Input: dimensioned drawing with shaded views. Units: mm. Origin: part minimum x, y, z. A direction names the side the tool comes from. Round coordinates to 2 decimals unless told otherwise and drop trailing zeros. Write each loop counter-clockwise with the first axis right and the second up, starting at its lowest first coordinate (ties: lowest second). Pieces come first, ordered by that corner, then holes. Notation, with made-up numbers: M 36,28 L 87,28 A12 cw 87,45 Z; hole C 22.5,63.5 d3. An arc over 180 degrees is marked long. Answer in a Markdown table with one row per item. Add a question column.
Item 1: Cut plane C-C on y = 2.25. Return loops of the section in (x, z), and give its area (3 significant figures).
Item 2: Mould query, pull axis Z, two halves, no side actions, for the marked faces 1, 2 and 3. Classes: released by +Z, released by -Z, zero draft, split by the parting line, or undercut.
Item 3: Cut plane A-A on z = 10. Return loops of the section in (x, y).
Item 4: Cut plane D-D on x = 12.5. Return loops of the section in (y, z).
Item 5: Set-up query: the marked faces 4 and 5. Return all of +Z, -Z, +X, -X, +Y, -Y with unobstructed straight access to the full face (end or side cutting, diameter ignored); none if empty.
Item 6: Cut plane B-B on x = 10. Return loops of the section in (y, z).
Item 7: Contact query for a flat-ended pin moving along its axis: pin 1 (2 mm diameter, centred on x = 14.5, z = 15, fed in from +Y). Output: stop coordinate, or through.
Item 8: Material intervals for probe 1 along X at (y, z) = (0.7, 10); probe 2 along X at (y, z) = (3.25, 6.75); probe 3 along Y at (x, z) = (8.25, 5.75), sorted ascending.
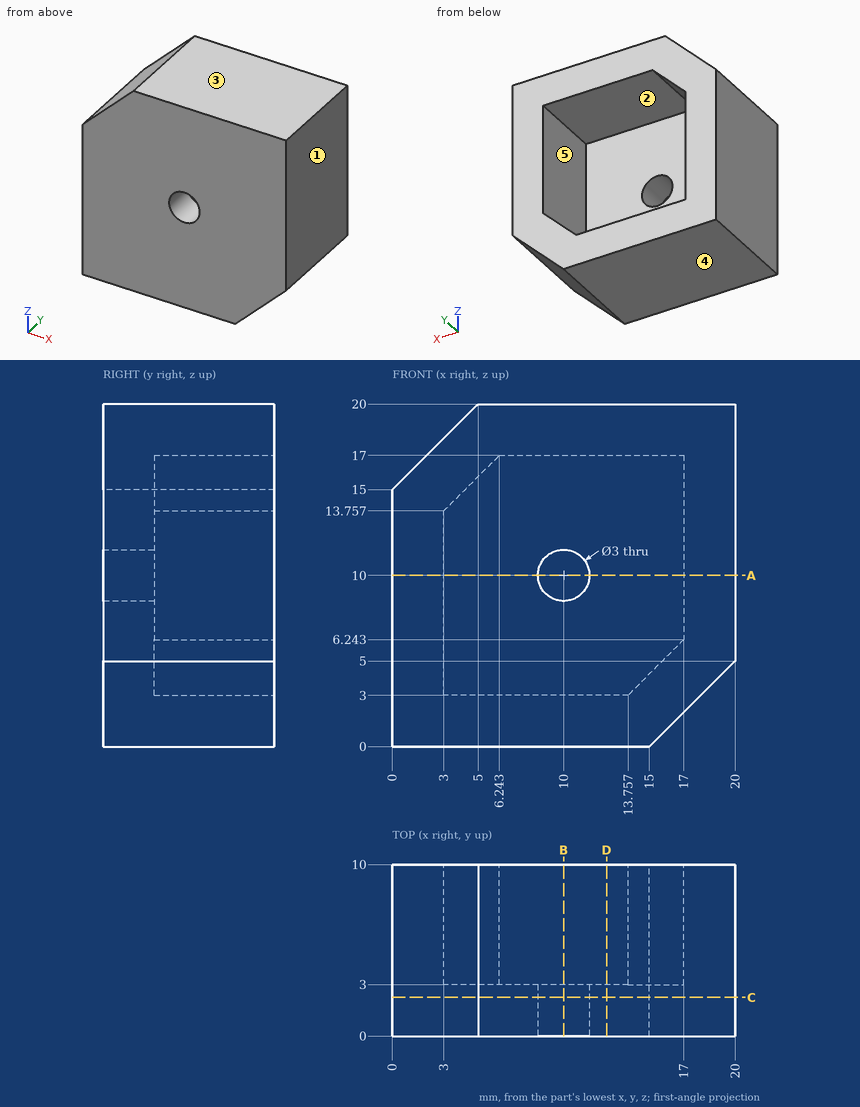
Results below:
| question | item | result |
|---|---|---|
| 1 | outline | M 0,0 L 15,0 L 20,5 L 20,20 L 5,20 L 0,15 Z; hole C 10,10 d3 |
| 1 | area | 368 mm2 |
| 2 | face 1 | zero draft |
| 2 | face 2 | undercut |
| 2 | face 3 | released by +Z |
| 3 | outline | M 0,0 L 8.5,0 L 8.5,3 L 3,3 L 3,10 L 0,10 Z; M 11.5,0 L 20,0 L 20,10 L 17,10 L 17,3 L 11.5,3 Z |
| 4 | outline | M 0,0 L 10,0 L 10,3 L 3,3 L 3,17 L 10,17 L 10,20 L 0,20 Z |
| 5 | face 4 | -Z, +X, -X, +Y, -Y |
| 5 | face 5 | +Y |
| 6 | outline | M 0,0 L 10,0 L 10,3 L 3,3 L 3,8.5 L 0,8.5 Z; M 0,11.5 L 3,11.5 L 3,17 L 10,17 L 10,20 L 0,20 Z |
| 7 | pin 1 | y = 3 |
| 8 | probe 1 | 0 to 8.5, 11.5 to 20 |
| 8 | probe 2 | 0 to 3, 17 to 20 |
| 8 | probe 3 | 0 to 3 |
